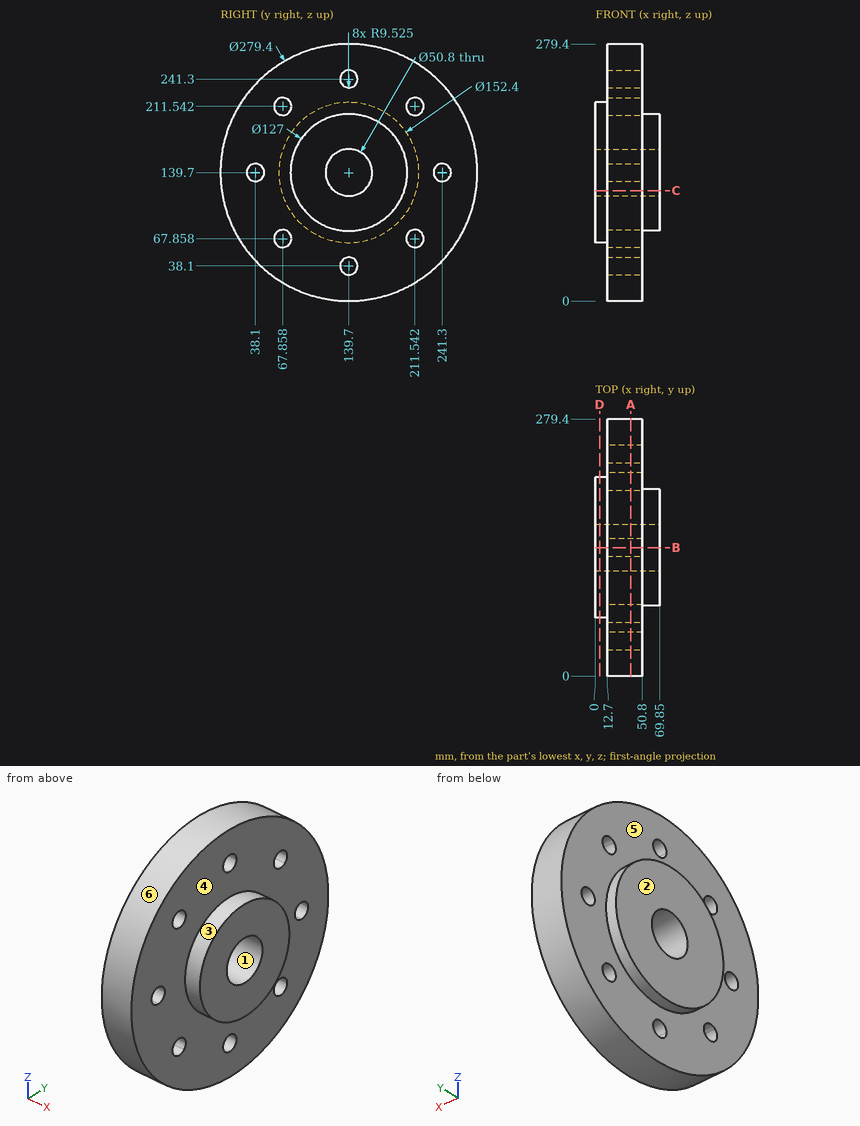
Input: dimensioned drawing with shaded views. Units: mm. Origin: part minimum x, y, z. A direction names the side the tool comes from. Round coordinates to 2 decimals unless told otherwise and drop trailing zeros. Loops run counter-clockwise (first coordinate to the right, second up) from the corner with the lowest first, then second, coordinate; pieces in that order, holes last. Notation, with made-up numbers: M 27.25,-11 L 85.25,-11 A32 ccw 85.25,22 Z; hole C 87,-33 d8. An arc over 180 degrees is marked long. Answer in a Markdown table with one row per item. Add a question column.
1. Mould query, pull axis Y, two halves, no side actions, for the marked faces 1, 2 and 3. Classes: released by +Y, released by -Y, zero draft, split by the parting line, or undercut.
2. Section B-B (y = 139.7). Output: boundary loops of the cut face in (x, z) (3 decimals).
3. Contact query for flat-ended pins moving along their axis: pin 1 (4 mm diameter, centred on x = 31, z = 173, fed in from -Y); pin 2 (4 mm diameter, centred on x = 52, y = 29, fed in from -Z); pin 3 (5 mm diameter, centred on y = 195.5, z = 229.5, fed in from +X). Output: stop coordinate, or through.
4. Section D-D (x = 4.5). Output: boundary loops of the cut face in (y, z).
5. Ray query, probe 1 along Y at (x, z) = (44.5, 139.7) (3 decimals); probe 2 along Z at (x, y) = (15, 139); probe 3 along Z at (x, y) = (25.5, 69). Return the intervals inside material, ascending.
6. Section C-C (z = 120). Output: boundary loops of the cut face in (x, y).
7. Section A-A (x = 38.5). Give the number of separate pieces and of enclosed holes in the cut face, and give its area (3 significant figures).
8. Set-up query: the marked faces 4, 5 and 6. Return all of +Z, -Z, +X, -X, +Y, -Y with unobstructed straight access to the full face (end or side cutting, diameter ignored); none if empty.
Values follow:
| question | item | result |
|---|---|---|
| 1 | face 1 | undercut |
| 1 | face 2 | zero draft |
| 1 | face 3 | split by the parting line |
| 2 | outline | M 0,63.5 L 12.7,63.5 L 12.7,47.625 L 50.8,47.625 L 50.8,76.2 L 69.85,76.2 L 69.85,114.3 L 0,114.3 Z; M 0,165.1 L 69.85,165.1 L 69.85,203.2 L 50.8,203.2 L 50.8,231.775 L 12.7,231.775 L 12.7,215.9 L 0,215.9 Z; M 12.7,0 L 50.8,0 L 50.8,28.575 L 12.7,28.575 Z; M 12.7,250.825 L 50.8,250.825 L 50.8,279.4 L 12.7,279.4 Z |
| 3 | pin 1 | y = 3.55 |
| 3 | pin 2 | z = 52.45 |
| 3 | pin 3 | x = 50.8 |
| 4 | outline | C 139.7,139.7 d152.4; hole C 139.7,139.7 d50.8 |
| 5 | probe 1 | 0 to 28.575, 47.625 to 114.3, 165.1 to 231.775, 250.825 to 279.4 |
| 5 | probe 2 | 0 to 28.6, 47.6 to 114.31, 165.09 to 231.8, 250.8 to 279.4 |
| 5 | probe 3 | 19.21 to 58.4, 77.31 to 202.09, 221 to 260.19 |
| 6 | outline | M 0,66.09 L 12.7,66.09 L 12.7,1.4 L 50.8,1.4 L 50.8,79.33 L 69.85,79.33 L 69.85,123.67 L 0,123.67 Z; M 0,155.73 L 69.85,155.73 L 69.85,200.07 L 50.8,200.07 L 50.8,278 L 12.7,278 L 12.7,213.31 L 0,213.31 Z |
| 7 | separate pieces | 1 |
| 7 | enclosed holes | 9 |
| 7 | area | 57,000 mm^2 |
| 8 | face 4 | +X |
| 8 | face 5 | -X |
| 8 | face 6 | +X, -X |
